Build history of the part. All positions in model axes, mm. A direction names the side the tool comes from. Give positions to 0.01 mm unless a question says otherwise; leave off trailing zeros. Write each loop counter-clockwise with the first axis right and the second up, starting at its lowest first coordinate (ties: lowest second). Pieces come first, ordered by that corner, then holes. Notation, with made-up numbers: (47.25, 77.25) - (59.25, 77.25) arc R30 cw to (59.25, 104.25) - close; hole circle Ø5 at (33.25, 45). An arc over 180 degrees is marked (long way). Use one line per item in the form item = value. Start each with the question number.
from build123d import *

# Parameters (mm, degrees)
SKETCH1_R           = 3.175
SKETCH1_R_2         = 2
SKETCH1_W           = 8
SKETCH1_H           = 5
BOSS_EXTRUDE1_DEPTH = 1.5875


with BuildPart() as part:
    # Sketch1 → Boss-Extrude1 (new body, symmetric)
    with BuildSketch(Plane(origin=(0, 0, 0), x_dir=(1, 0, 0), z_dir=(0, 1, 0))):
        with BuildLine():
            Line((22.225, 0), (22.225, -250.448449629))
            ThreePointArc((22.225, -250.448449629), (23.079031542, -256.245526228), (25.568559237, -261.550026094))
            Line((25.568559237, -261.550026094), (14.961957519, -272.156627812))
            Line((14.961957519, -272.156627812), (20.618811769, -277.813482061))
            Line((20.618811769, -277.813482061), (31.225413487, -267.206880343))
            ThreePointArc((31.225413487, -267.206880343), (42.326989951, -270.55043958), (53.428566416, -267.206880343))
            Line((53.428566416, -267.206880343), (64.035168134, -277.813482061))
            Line((64.035168134, -277.813482061), (69.692022383, -272.156627812))
            Line((69.692022383, -272.156627812), (59.085420665, -261.550026094))
            ThreePointArc((59.085420665, -261.550026094), (60.653609073, -258.708294153), (61.744021205, -255.651227473))
            Line((61.744021205, -255.651227473), (95.551425125, -264.709894052))
            ThreePointArc((95.551425125, -264.709894052), (36.163593878, -305.204653346), (-12.736009339, -252.520985708))
            Line((-12.736009339, -252.520985708), (-22.209273391, -0.835942847))
            ThreePointArc((-22.209273391, -0.835942847), (-14.554726567, 16.796147164), (3.986980194, 21.864460065))
            Line((3.986980194, 21.864460065), (11.70043151, 31.056993382))
            Line((11.70043151, 31.056993382), (28.553409259, 16.915665969))
            Line((28.553409259, 16.915665969), (20.839957942, 7.723132652))
            ThreePointArc((20.839957942, 7.723132652), (21.875999295, 3.923172169), (22.225, 0))
        make_face()
        Circle(SKETCH1_R, mode=Mode.SUBTRACT)
        with Locations((16.270194726, 19.390063017)):
            Circle(SKETCH1_R_2, mode=Mode.SUBTRACT)
        with Locations((-11, 0)):
            Rectangle(SKETCH1_W, SKETCH1_H, mode=Mode.SUBTRACT)
    extrude(amount=BOSS_EXTRUDE1_DEPTH, both=True)


solid = part.part
(1) Cut at A-A, the plane x = 0. Give the cut face in (y, z) (1 decimal).
(2) Which spindle directions (+Z, -Z, +X, -X, +Y, -Y) get a long thin tool onto all of the face, cutting with end or side? Do faces 1 (the flat face through (24.75, 0.02, -12.38)), 2 (the flat face through (66.824, 0.022, 275.025)), 3 (the flat face through (19, -1.588, 161)). Say none if no direction does.
(3) Pin check, flat tip, straight feed: pin 1 Ø1.6 at (y, z) = (-0.5, -1) entering from +X. Stop position of the tip, or through.
(4) Cut at C-C, the plane z = 157.5. Give the cut face in (x, y) (1 decimal), then the cut area to 3 significant figures.
(5) Cut at D-D, the plane z = 116.5. Give the cut face in (x, y) (1 decimal), then the cut area to 3 significant figures.
(6) Cut at B-B, the plane y = -0.25. Give the cut face in (x, z) (3 decimals).
(7) Two-plate mould, pull along Z, no slides. Class faces 4 (the flat face through (20.009, 0.022, -24.085)), 5 (the flat face through (-17.406, 0.022, 128.44)), 6 (the flat face through (17.751, 0.022, 274.945)): +Z half, -Z half, draft (parallel to the pull), parting line (faces both ways), or undercut.
(8) Wall check: line 1 (X direction, y = 1.2, z = -2); line 2 (X direction, y = 0, z = 274); line 3 (Z direction, x = 17, y = -0.3). Give the ranges that are in metal, low to high. Write a range as from..to.
Solution:
q1.outline = (-1.6, -22.2) - (1.6, -22.2) - (1.6, -3.2) - (-1.6, -3.2) - close; (-1.6, 3.2) - (1.6, 3.2) - (1.6, 285.7) - (-1.6, 285.7) - close
q2.face_1 = +X, +Y, -Y
q2.face_2 = +Y, -Y
q2.face_3 = +Z, -Z, +X, -X, -Y
q3.pin_1 = 22.22
q4.outline = (-16.3, -1.6) - (22.2, -1.6) - (22.2, 1.6) - (-16.3, 1.6) - close
q4.area = 122 mm2
q5.outline = (-17.9, -1.6) - (22.2, -1.6) - (22.2, 1.6) - (-17.9, 1.6) - close
q5.area = 127 mm2
q6.outline = (-22.209, 0.836) arc R22.225 ccw to (3.987, -21.864) - (11.7, -31.057) - (28.553, -16.916) - (20.84, -7.723) arc R22.225 ccw to (22.225, 0) - (22.225, 250.448) arc R20.102 cw to (25.569, 261.55) - (14.962, 272.157) - (20.619, 277.813) - (31.225, 267.207) arc R20.102 cw to (53.429, 267.207) - (64.035, 277.813) - (69.692, 272.157) - (59.085, 261.55) arc R20.102 cw to (61.744, 255.651) - (95.551, 264.71) arc R55.102 ccw to (-12.736, 252.521) - close; hole (-15, -2.5) - (-7, -2.5) - (-7, 2.5) - (-15, 2.5) - close; hole circle Ø6.35 at (0, 0); hole circle Ø4 at (16.27, -19.39)
q7.face_4 = -Z half
q7.face_5 = +Z half
q7.face_6 = undercut
q8.line_1 = -22.13..-15, -7..-2.47, 2.47..22.13
q8.line_2 = -7.49..16.81, 24.43..60.22, 67.85..92.14
q8.line_3 = -26.61..-21.25, -17.53..270.12, 274.19..299.38
